Check sheet for the modelled part. Datum: model origin and axes. Units: mm. A direction names the side the tool comes from. Coordinates: 2 decimals unless noted, no trailing zeros. Write each loop counter-clockwise with the first axis right and the second up, starting at its lowest first coordinate (ties: lowest second). Pieces come first, ordered by that corner, then holes. Notation, with made-up numbers: M -29,2 L -22,2 A21 ccw -22,8 Z; hole C 3,-0.75 d5. An arc over 180 degrees is marked long. Answer as CSV lines item,"result".
from build123d import *

# Parameters (mm, degrees)
F1_DEPTH = 10
F2_R     = 3.275
F3_DEPTH = 13.1418462065
F4_R     = 3
F5_R     = 8


with BuildPart() as f1:
    # F0 (on Top) → F1 (new body, symmetric)
    with BuildSketch(Plane.XY):
        with BuildLine():
            Line((11.1408462065, 6.968743418), (11.1408462065, 0))
            ThreePointArc((11.1408462065, 0), (-7.8777679008, -7.8777679008), (0, 11.1408462065))
            Line((0, 11.1408462065), (6.968743418, 11.1408462065))
            ThreePointArc((6.968743418, 11.1408462065), (3.6250305111, 12.6309537572), (0, 13.1408462065))
            ThreePointArc((0, 13.1408462065), (-9.2919814631, -9.2919814631), (13.1408462065, 0))
            ThreePointArc((13.1408462065, 0), (12.6309537572, 3.6250305111), (11.1408462065, 6.968743418))
        make_face()
        with BuildLine():
            ThreePointArc((0, 13.1408462065), (3.6250305111, 12.6309537572), (6.968743418, 11.1408462065))
            Line((6.968743418, 11.1408462065), (9.1408462065, 11.1408462065))
            Line((9.1408462065, 11.1408462065), (9.1408462065, 33.1408462065))
            Line((9.1408462065, 33.1408462065), (7.1408462065, 33.1408462065))
            Line((7.1408462065, 33.1408462065), (7.1408462065, 13.1408462065))
            Line((7.1408462065, 13.1408462065), (0, 13.1408462065))
        make_face()
        with BuildLine():
            Line((11.1408462065, 33.1408462065), (11.1408462065, 6.968743418))
            ThreePointArc((11.1408462065, 6.968743418), (12.6309537572, 3.6250305111), (13.1408462065, 0))
            Line((13.1408462065, 0), (13.1408462065, 33.1408462065))
            Line((13.1408462065, 33.1408462065), (11.1408462065, 33.1408462065))
        make_face()
    extrude(amount=F1_DEPTH, both=True)

    # F2 (on Right) → F3 (cut, through all)
    with BuildSketch(Plane.YZ):
        with Locations((23.1408462065, 0)):
            Circle(F2_R)
    extrude(amount=F3_DEPTH, mode=Mode.SUBTRACT)

    # F4
    f4_edges = [f1.edges().sort_by_distance(p)[0] for p in [
        (7.140846, 13.140846, 0),
    ]]
    fillet(f4_edges, radius=F4_R)

    # F5
    f5_edges = [f1.edges().sort_by_distance(p)[0] for p in [
        (8.140846, 33.140846, 10),
        (12.140846, 33.140846, 10),
        (12.140846, 33.140846, -10),
        (8.140846, 33.140846, -10),
    ]]
    fillet(f5_edges, radius=F5_R)


solid = f1.part
1) Section check C-C, the plane x = 7.75. Give the number of separate pieces and of enclosed holes in the cut face, plus the area to 3 significant figures.
Answer key:
separate pieces,"2"
enclosed holes,"1"
area,"431 mm2"
2) Section check A-A, the plane y = 17. Record the boundary of the cut face in (x, z), plus the area to 3 significant figures.
Answer key:
outline,"M 7.14,-10 L 9.14,-10 L 9.14,10 L 7.14,10 Z; M 11.14,-10 L 13.14,-10 L 13.14,10 L 11.14,10 Z"
area,"80.0 mm2"
3) Section check D-D, the plane x = 2. Record the boundary of the cut face in (y, z).
Answer key:
outline,"M -12.99,-10 L -10.96,-10 L -10.96,10 L -12.99,10 Z; M 11.14,-10 L 13.14,-10 L 13.14,10 L 11.14,10 Z"
4) Section check B-B, the plane z = 0. Record the boundary of the cut face in (x, y).
Answer key:
outline,"M 0,11.14 L 9.14,11.14 L 9.14,19.87 L 7.14,19.87 L 7.14,16.14 A3 cw 4.14,13.14 L 0,13.14 A13.14 ccw long 13.14,0 L 13.14,19.87 L 11.14,19.87 L 11.14,0 A11.14 cw long Z; M 7.14,26.42 L 9.14,26.42 L 9.14,33.14 L 7.14,33.14 Z; M 11.14,26.42 L 13.14,26.42 L 13.14,33.14 L 11.14,33.14 Z"
5) Tool access check on faces 1 (the face through (9.141, 19.5, 0.1)), 2 (the face through (5, 11.141, 0)), 3 (the face through (3, 12, -10)), 4 (the face through (2, 13.141, 0)). Record the directions out of +Z, -Z, +X, -X, +Y, -Y that give a thin tool (end or side, any length) a straight path to the whole face; none if there is none.
Answer key:
face 1,"+Z, -Z, +Y"
face 2,"+Z, -Z"
face 3,"-Z, +X, -X, +Y, -Y"
face 4,"+Z, -Z, -X, +Y"
6) Depth check by flat-ended pin: P1, Ø8.5, axis at y = 23.5, z = -1.5, coming from the -X side; P2, Ø6, axis at y = 23.14, z = 0, coming from the +X side; P3, Ø3.5, axis at x = 2.5, z = -3, coming from the +Y side; P4, Ø1, axis at x = 5, z = 6.5, coming from the -Y side. Enter the tip coordinate at first touch or a pass-through.
Answer key:
P1,"stops at x = 7.14"
P2,"passes through"
P3,"stops at y = 13.14"
P4,"stops at y = -12.35"
7) Thickness scan on line 1 along X through (y, z) = (22, 4.75); line 2 along X through (y, z) = (0, -2.75); line 3 along Y through (x, z) = (8.5, 0). Record the ranges inside material, lowest first.
Answer key:
line 1,"x = 7.14 to 9.14, 11.14 to 13.14"
line 2,"x = -13.14 to -11.14, 11.14 to 13.14"
line 3,"y = -10.02 to -7.2, 11.14 to 19.87, 26.42 to 33.14"
8) Mould release check, pull along X, two halves, no side actions. Record for faces 5 (the face through (12.127, 26.265, 0.984)), 6 (the face through (11.141, 17, 0)), 7 (the face through (7.141, 27, 0)): pulls with the +X half, pulls with the -X half, needs draft (parallel to the pull), parting line crosses it, or undercut.
Answer key:
face 5,"needs draft"
face 6,"undercut"
face 7,"pulls with the -X half"
